Read the model definition and answer for the solid it produces. Units are mm, in the model's axes. Coordinates: 2 decimals unless noted, no trailing zeros. Write each loop counter-clockwise with the first axis right and the second up, starting at its lowest first coordinate (ties: lowest second). Pieces come first, ordered by that corner, then holes.
from build123d import *

# Parameters (mm, degrees)
SKETCH1_R           = 1.175
SKETCH1_R_2         = 1.55
BOSS_EXTRUDE1_DEPTH = 3.175
CUT_EXTRUDE2_DEPTH  = 4.175
CUT_EXTRUDE1_DEPTH  = 4.175
CIRPATTERN1_COUNT   = 4
CHAMFER1_SIZE       = 1.7


with BuildPart() as part:
    # Sketch1 → Boss-Extrude1 (new body)
    with BuildSketch(Plane.XY):
        with BuildLine():
            ThreePointArc((-28.274738921, -34.524335822), (-25.595848472, -36.554659976), (-22.771733351, -38.377581805))
            ThreePointArc((-22.771733351, -38.377581805), (-1.930585195, -44.583219554), (19.368987874, -40.202399602))
            ThreePointArc((19.368987874, -40.202399602), (22.3125, -38.646383644), (25.131805412, -36.875235345))
            ThreePointArc((25.131805412, -36.875235345), (42.197997698, -14.516184597), (42.498870951, 13.610165056))
            ThreePointArc((42.498870951, 13.610165056), (41.827558264, 15.551398481), (41.067627867, 17.459684027))
            ThreePointArc((41.067627867, 17.459684027), (25.603337609, 36.549414883), (2.379040875, 44.561539353))
            ThreePointArc((2.379040875, 44.561539353), (0, 44.625), (-2.379040875, 44.561539353))
            ThreePointArc((-2.379040875, 44.561539353), (-42.409403049, 13.886437917), (-28.274738921, -34.524335822))
        make_face()
        with Locations((-26, -26)):
            Circle(SKETCH1_R, mode=Mode.SUBTRACT)
        with Locations((0, -22)):
            Circle(SKETCH1_R_2, mode=Mode.SUBTRACT)
        with Locations((-22, 0)):
            Circle(SKETCH1_R_2, mode=Mode.SUBTRACT)
        with BuildLine():
            ThreePointArc((-7.14068763, 16.283088778), (-4.469980501, 16.914656425), (-1.748739828, 16.559123782))
            ThreePointArc((-1.748739828, 16.559123782), (0, 16.285), (1.748739828, 16.559123782))
            ThreePointArc((1.748739828, 16.559123782), (4.469980501, 16.914656425), (7.14068763, 16.283088778))
            ThreePointArc((7.14068763, 16.283088778), (12.572358569, 12.572358569), (16.283088778, 7.14068763))
            ThreePointArc((16.283088778, 7.14068763), (16.914656425, 4.469980501), (16.559123782, 1.748739828))
            ThreePointArc((16.559123782, 1.748739828), (16.285, 0), (16.559123782, -1.748739828))
            ThreePointArc((16.559123782, -1.748739828), (16.914656425, -4.469980501), (16.283088778, -7.14068763))
            ThreePointArc((16.283088778, -7.14068763), (12.572358569, -12.572358569), (7.14068763, -16.283088778))
            ThreePointArc((7.14068763, -16.283088778), (4.469980501, -16.914656425), (1.748739828, -16.559123782))
            ThreePointArc((1.748739828, -16.559123782), (0, -16.285), (-1.748739828, -16.559123782))
            ThreePointArc((-1.748739828, -16.559123782), (-4.469980501, -16.914656425), (-7.14068763, -16.283088778))
            ThreePointArc((-7.14068763, -16.283088778), (-12.572358569, -12.572358569), (-16.283088778, -7.14068763))
            ThreePointArc((-16.283088778, -7.14068763), (-16.914656425, -4.469980501), (-16.559123782, -1.748739828))
            ThreePointArc((-16.559123782, -1.748739828), (-16.285, 0), (-16.559123782, 1.748739828))
            ThreePointArc((-16.559123782, 1.748739828), (-16.914656425, 4.469980501), (-16.283088778, 7.14068763))
            ThreePointArc((-16.283088778, 7.14068763), (-12.572358569, 12.572358569), (-7.14068763, 16.283088778))
        make_face(mode=Mode.SUBTRACT)
        with Locations((26, -26)):
            Circle(SKETCH1_R, mode=Mode.SUBTRACT)
        with Locations((22, 0)):
            Circle(SKETCH1_R_2, mode=Mode.SUBTRACT)
        with Locations((0, 22)):
            Circle(SKETCH1_R_2, mode=Mode.SUBTRACT)
        with Locations((-26, 26)):
            Circle(SKETCH1_R, mode=Mode.SUBTRACT)
        with Locations((26, 26)):
            Circle(SKETCH1_R, mode=Mode.SUBTRACT)
    extrude(amount=BOSS_EXTRUDE1_DEPTH)

    # Sketch3 → Cut-Extrude2 (cut, through all)
    with BuildSketch(Plane.XY.offset(3.175)):
        with BuildLine():
            ThreePointArc((-32.152970188, 30.944743222), (-34.933731714, 27.767337171), (-37.401738142, 24.341335398))
            Line((-37.401738142, 24.341335398), (-32.152970188, 24.341335398))
            Line((-32.152970188, 24.341335398), (-32.152970188, 30.944743222))
        make_face()
        with BuildLine():
            Line((-32.152970188, -24.341335398), (-37.401738142, -24.341335398))
            ThreePointArc((-37.401738142, -24.341335398), (-34.933731714, -27.767337171), (-32.152970188, -30.944743222))
            Line((-32.152970188, -30.944743222), (-32.152970188, -24.341335398))
        make_face()
        with BuildLine():
            ThreePointArc((-24.341335398, 37.401738142), (-27.767337171, 34.933731714), (-30.944743222, 32.152970188))
            Line((-30.944743222, 32.152970188), (-24.341335398, 32.152970188))
            Line((-24.341335398, 32.152970188), (-24.341335398, 37.401738142))
        make_face()
        with BuildLine():
            ThreePointArc((30.944743222, 32.152970188), (27.767337171, 34.933731714), (24.341335398, 37.401738142))
            Line((24.341335398, 37.401738142), (24.341335398, 32.152970188))
            Line((24.341335398, 32.152970188), (30.944743222, 32.152970188))
        make_face()
        with BuildLine():
            Line((-24.341335398, -32.152970188), (-30.944743222, -32.152970188))
            ThreePointArc((-30.944743222, -32.152970188), (-27.767337171, -34.933731714), (-24.341335398, -37.401738142))
            Line((-24.341335398, -37.401738142), (-24.341335398, -32.152970188))
        make_face()
        with BuildLine():
            ThreePointArc((37.401738142, 24.341335398), (34.933731714, 27.767337171), (32.152970188, 30.944743222))
            Line((32.152970188, 30.944743222), (32.152970188, 24.341335398))
            Line((32.152970188, 24.341335398), (37.401738142, 24.341335398))
        make_face()
        with BuildLine():
            Line((24.341335398, -32.152970188), (24.341335398, -37.401738142))
            ThreePointArc((24.341335398, -37.401738142), (27.767337171, -34.933731714), (30.944743222, -32.152970188))
            Line((30.944743222, -32.152970188), (24.341335398, -32.152970188))
        make_face()
        with BuildLine():
            Line((32.152970188, -24.341335398), (32.152970188, -30.944743222))
            ThreePointArc((32.152970188, -30.944743222), (34.933731714, -27.767337171), (37.401738142, -24.341335398))
            Line((37.401738142, -24.341335398), (32.152970188, -24.341335398))
        make_face()
    extrude(amount=-CUT_EXTRUDE2_DEPTH, mode=Mode.SUBTRACT)

    # Sketch2 → Cut-Extrude1 (cut, through all)
    with BuildSketch(Plane.XY.offset(3.175)):
        with BuildLine():
            Line((-16.518713095, 28.611250357), (-15.76028553, 27.29761528))
            ThreePointArc((-15.76028553, 27.29761528), (-13.666256903, 25.588365448), (-10.965441293, 25.698301447))
            ThreePointArc((-10.965441293, 25.698301447), (0, 27.94), (10.965441293, 25.698301447))
            ThreePointArc((10.965441293, 25.698301447), (13.666256903, 25.588365448), (15.76028553, 27.29761528))
            Line((15.76028553, 27.29761528), (16.518713095, 28.611250357))
            ThreePointArc((16.518713095, 28.611250357), (16.929410685, 33.153177065), (13.732973771, 36.405954615))
            ThreePointArc((13.732973771, 36.405954615), (0, 38.91), (-13.732973771, 36.405954615))
            ThreePointArc((-13.732973771, 36.405954615), (-16.929410685, 33.153177065), (-16.518713095, 28.611250357))
        make_face()
    cut_extrude1 = extrude(amount=-CUT_EXTRUDE1_DEPTH, mode=Mode.SUBTRACT)

    # CirPattern1: Cut-Extrude1 ×4 about axis
    cirpattern1_axis = Axis((0, 0, 0), (0, 0, 1))
    for i in range(1, CIRPATTERN1_COUNT):
        add(cut_extrude1.rotate(cirpattern1_axis, i * 360 / CIRPATTERN1_COUNT), mode=Mode.SUBTRACT)

    # Chamfer1
    chamfer1_edges = [part.edges().sort_by_distance(p)[0] for p in [
        (20.45, 0, 3.175),
        (-1.55, -22, 3.175),
        (-23.55, 0, 3.175),
        (-1.55, 22, 3.175),
    ]]
    chamfer(chamfer1_edges, length=CHAMFER1_SIZE)


solid = part.part
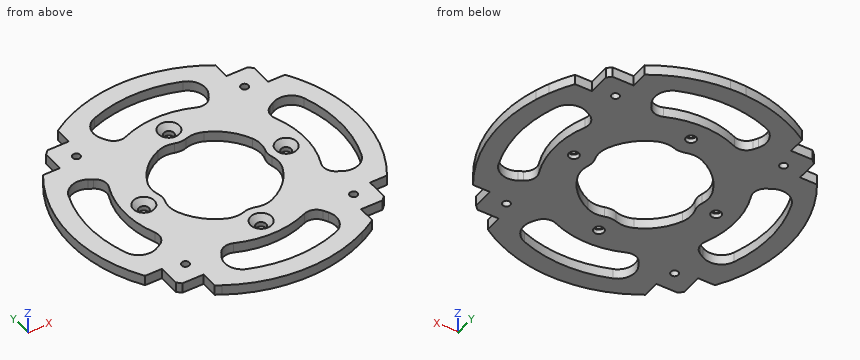
Item 1: The part is cut by section C-C (x = 22). Give the vertices of the cut face in (y, z) (3 decimals), and give its area (3 significant figures).
Item 2: Find the intervals of material crossed by probe 1 along Y at (x, z) = (0, 0.6) (3 decimals); probe 2 along Y at (x, z) = (-4.5, 1.25); probe 3 along Y at (x, z) = (9.5, 2.85), in increasing order.
Item 3: The part is cut by section A-A (y = 0). Give the vertices of the cut face in (x, z) (3 decimals), and give its area (3 significant figures).
Item 4: The part is cut by section D-D (z = 2.1). State how many separate pieces and enclosed holes the cut face has, and give its area (3 significant figures).
Item 5: Given pin 1 (1 mm diameter, centred on y = -34, z = 1, fed in from +X); pin 2 (1.6 mm diameter, centred on x = 34.5, z = 1, fed in from -Y); pin 3 (1.9 mm diameter, centred on x = 26, y = 26, fed in from +Z); pin 4 (1.6 mm diameter, centred on x = 29, z = 2, fed in from -Y), each flat-ended and moving along its own axis, determine where each tip first touches the part or whether it passes through.
Answer:
1. outline: (-38.825, 0) - (-1.55, 0) - (-1.55, 1.475) - (-3.25, 3.175) - (-38.825, 3.175) - close; (1.55, 0) - (38.825, 0) - (38.825, 3.175) - (3.25, 3.175) - (1.55, 1.475) - close
1. area: 234 mm2
2. probe 1: y = -44.625 to -38.91, -27.94 to -23.55, -20.45 to -16.285, 16.285 to 20.45, 23.55 to 27.94, 38.91 to 44.625
2. probe 2: y = -44.4 to -38.65, -27.58 to -16.91, 16.91 to 27.58, 38.65 to 44.4
2. probe 3: y = -43.6 to -37.73, -26.28 to -15.03, 15.03 to 26.28, 37.73 to 43.6
3. outline: (-44.625, 0) - (-38.91, 0) - (-38.91, 3.175) - (-44.625, 3.175) - close; (-27.94, 0) - (-23.55, 0) - (-23.55, 1.475) - (-25.25, 3.175) - (-27.94, 3.175) - close; (-20.45, 0) - (-16.285, 0) - (-16.285, 3.175) - (-18.75, 3.175) - (-20.45, 1.475) - close; (16.285, 0) - (20.45, 0) - (20.45, 1.475) - (18.75, 3.175) - (16.285, 3.175) - close; (23.55, 0) - (27.94, 0) - (27.94, 3.175) - (25.25, 3.175) - (23.55, 1.475) - close; (38.91, 0) - (44.625, 0) - (44.625, 3.175) - (38.91, 3.175) - close
3. area: 84.8 mm2
4. separate pieces: 1
4. enclosed holes: 13
4. area: 3,620 mm2
5. pin 1: stops at x = 24.34
5. pin 2: stops at y = -24.34
5. pin 3: passes through
5. pin 4: stops at y = -32.15
